from build123d import *

# Parameters (mm, degrees)
F2_R     = 2.99
F3_DEPTH = 20


with BuildPart() as f1:
    # F0 (on Front) → F1 (revolve)
    with BuildSketch(Plane.XZ):
        Polygon((-17.5, 0), (0, 0), (0, 5.283122), (-12.5, 12.5), (-12.5, 30), (-17.5, 30), (-17.5, 16.6), (-15.05, 16.6), (-15.05, 13.5), (-17.5, 13.5), (-17.5, 6.6), (-15.05, 6.6), (-15.05, 3.5), (-17.5, 3.5), align=None)
    revolve(axis=Axis((0, 0, 2.641561), (0, 0, 1)))

    # F2 (on Front) → F3 (cut, symmetric)
    with BuildSketch(Plane.XZ):
        with Locations((0, 22)):
            Circle(F2_R)
    extrude(amount=F3_DEPTH, both=True, mode=Mode.SUBTRACT)


solid = f1.part
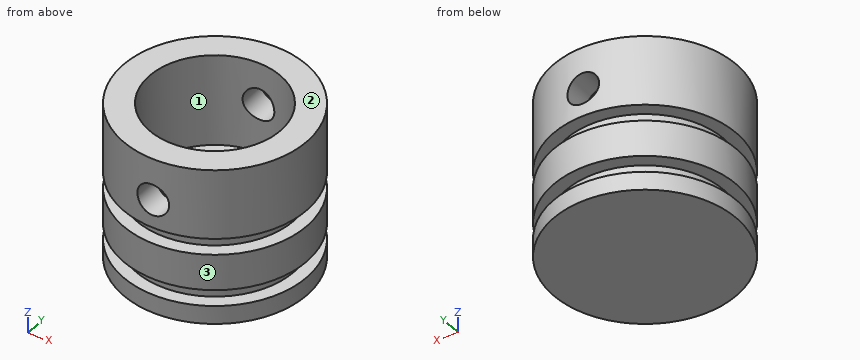
CAD build for the part. Positions are in the model's coordinates, mm. Face numbers are marked on the shaded views. Coordinates: 2 decimals unless noted, no trailing zeros. Loops run counter-clockwise (first coordinate to the right, second up) from the corner with the lowest first, then second, coordinate; pieces in that order, holes last. Notation, with made-up numbers: (79.25, 21) -> (111.25, 21) arc R16 cw to (111.25, 40) -> close; hole circle Ø11 at (29.5, -31.75). An arc over 180 degrees is marked (long way). One line per item, written item: value.
1. Slice it at C-C on x = 14.5. Write the cut outline in (y, z).
Answers:
outline: (-9.8, 0) -> (9.8, 0) -> (9.8, 3.5) -> (4.03, 3.5) -> (4.03, 6.6) -> (9.8, 6.6) -> (9.8, 13.5) -> (4.03, 13.5) -> (4.03, 16.6) -> (9.8, 16.6) -> (9.8, 30) -> (-9.8, 30) -> (-9.8, 16.6) -> (-4.03, 16.6) -> (-4.03, 13.5) -> (-9.8, 13.5) -> (-9.8, 6.6) -> (-4.03, 6.6) -> (-4.03, 3.5) -> (-9.8, 3.5) -> close
2. Drill centre lines: line 1 (Z direction, x = 0, y = -14); line 2 (X direction, y = 0, z = 24); line 3 (X direction, y = 14.45, z = 22). Where is each one in solid material? Low to high. Write a range as [from, to].
Answers:
line 1: z = [0, 19.01], [24.99, 30]
line 2: x = [-17.5, -12.5], [12.5, 17.5]
line 3: x = [-9.87, -2.99], [2.99, 9.87]
3. Pull direction X, two halves, no side cores. Call the marked faces 1, 2 and 3: pulls with the +X half, pulls with the -X half, needs draft (parallel to the pull), parting line crosses it, or undercut.
Answers:
face 1: undercut
face 2: needs draft
face 3: parting line crosses it
4. Flat gauge pins, fed straight in: P1, Ø15, axis at x = 0, y = 0, coming from the +Z side; P2, Ø5, axis at y = -5.5, z = 20.5, coming from the -X side; P3, Ø2, axis at y = -2.5, z = 23.5, coming from the -X side. Where does each tip first touch, or does it go through?
Answers:
P1: stops at z = 9.61
P2: stops at x = -17.24
P3: stops at x = -17.44
5. Slice it at B-B on z = 18. Write the cut outline in (x, y), and give its area (3 significant figures).
Answers:
outline: circle Ø35 at (0, 0); hole circle Ø25 at (0, 0)
area: 471 mm^2
6. Slice it at A-A on z = 22. Write the cut outline in (x, y), and give its area (3 significant figures).
Answers:
outline: (-2.99, -17.24) -> (-2.99, -12.14) arc R12.5 cw to (-2.99, 12.14) -> (-2.99, 17.24) arc R17.5 ccw to start; (2.99, -17.24) arc R17.5 ccw to (2.99, 17.24) -> (2.99, 12.14) arc R12.5 cw to (2.99, -12.14) -> close
area: 411 mm^2
7. Slice it at D-D on z = 4.5. Write the cut outline in (x, y), and give its area (3 significant figures).
Answers:
outline: circle Ø30.1 at (0, 0)
area: 712 mm^2
